Here's how the part is built. I have some questions about the finished solid (model axes, mm). A direction names the side the tool comes from. Give positions to 0.01 mm unless a question says otherwise; leave off trailing zeros. Write each loop counter-clockwise with the first axis right and the second up, starting at its lowest first coordinate (ties: lowest second). Pieces come first, ordered by that corner, then holes. Notation, with made-up numbers: (46, 13) - (51, 13) arc R24 cw to (51, 27) - close; hole circle Ø11 at (48, 47.25). An arc over 180 degrees is marked (long way). Use a Markdown table: item, result.
```python
from build123d import *
from OCP.BRepFilletAPI import BRepFilletAPI_MakeChamfer

# Parameters (mm, degrees)
EXTRUDE_1_DEPTH   = 0.32
EXTRUDE_1_2_DEPTH = 0.32
CHAMFER_1_SIZE    = 0.1
CHAMFER_1_SIZE2   = 0.274747742
FILLET_1_R        = 0.5
CHAMFER_2_SIZE    = 0.1
CHAMFER_2_SIZE2   = 0.274747742
FILLET_2_R        = 0.5
SKETCH_2_W        = 2.54
SKETCH_2_H        = 5
EXTRUDE_2_DEPTH   = 1.8
CHAMFER_3_SIZE    = 0.5
CHAMFER_4_SIZE    = 0.25
EXTRUDE_3_DEPTH   = 0.7


with BuildPart() as part:
    # Sketch 1 → Extrude 1 (new, symmetric)
    with BuildSketch(Plane(origin=(0, 0, 0), x_dir=(0, 0, -1), z_dir=(1, 0, 0))):
        Polygon((-0.7385, 0), (0.7385, 0), (0.7385, 0.64), (-0.47340332, 0.64), (-1.38340332, 1.55), (-11.4615, 1.55), (-11.4615, 0.91), (-1.6485, 0.91), align=None)
    extrude(amount=EXTRUDE_1_DEPTH, both=True)

    # Chamfer 2: one chamfer whose edges measure the first distance from different faces: ONE call of the kernel's chamfer builder (chamfer() names one face for all edges)
    chamfer_2_edges_1 = [part.edges().sort_by_distance(p)[0] for p in [
        (0.32, 0.32, -0.7385),
        (0, 0, -0.7385),
        (0, 0.64, -0.7385),
        (-0.32, 0.32, -0.7385),
    ]]
    chamfer_2_side_1 = [part.faces().sort_by_distance(p)[0] for p in [
        (0, 0.32, -0.7385),
    ]]
    chamfer_2_edges_2 = [part.edges().sort_by_distance(p)[0] for p in [
        (0, 0.91, 11.4615),
        (0, 1.55, 11.4615),
        (-0.32, 1.23, 11.4615),
        (0.32, 1.23, 11.4615),
    ]]
    chamfer_2_side_2 = [part.faces().sort_by_distance(p)[0] for p in [
        (0, 1.23, 11.4615),
    ]]
    chamfer_2 = BRepFilletAPI_MakeChamfer(part.part.solid().wrapped)
    for e in chamfer_2_edges_1:
        chamfer_2.Add(CHAMFER_2_SIZE, CHAMFER_2_SIZE2, e.wrapped, chamfer_2_side_1[0].wrapped)  # the first distance lies on this face
    for e in chamfer_2_edges_2:
        chamfer_2.Add(CHAMFER_2_SIZE, CHAMFER_2_SIZE2, e.wrapped, chamfer_2_side_2[0].wrapped)  # the first distance lies on this face
    add(Compound.cast(chamfer_2.Shape()), mode=Mode.REPLACE)

    # Fillet 2
    fillet_2_edges = [part.edges().sort_by_distance(p)[0] for p in [
        (0, 0, 0.7385),
        (0, 0.91, 1.6485),
        (0, 1.55, 1.38340332),
        (0, 0.64, 0.47340332),
    ]]
    fillet(fillet_2_edges, radius=FILLET_2_R)



with BuildPart() as body_2:
    # Sketch 1 → Extrude 1 2 (new, symmetric)
    with BuildSketch(Plane(origin=(0, 0, 0), x_dir=(0, 0, -1), z_dir=(1, 0, 0))):
        Polygon((4.0615, 0), (5.5385, 0), (5.5385, 0.64), (4.32659668, 0.64), (0.87659668, 4.09), (-11.4615, 4.09), (-11.4615, 3.45), (0.6115, 3.45), align=None)
    extrude(amount=EXTRUDE_1_2_DEPTH, both=True)

    # Chamfer 1: one chamfer whose edges measure the first distance from different faces: ONE call of the kernel's chamfer builder (chamfer() names one face for all edges)
    chamfer_1_edges_1 = [body_2.edges().sort_by_distance(p)[0] for p in [
        (-0.32, 0.32, -5.5385),
        (0, 0.64, -5.5385),
        (0, 0, -5.5385),
        (0.32, 0.32, -5.5385),
    ]]
    chamfer_1_side_1 = [body_2.faces().sort_by_distance(p)[0] for p in [
        (0, 0.32, -5.5385),
    ]]
    chamfer_1_edges_2 = [body_2.edges().sort_by_distance(p)[0] for p in [
        (0, 3.45, 11.4615),
        (0, 4.09, 11.4615),
        (-0.32, 3.77, 11.4615),
        (0.32, 3.77, 11.4615),
    ]]
    chamfer_1_side_2 = [body_2.faces().sort_by_distance(p)[0] for p in [
        (0, 3.77, 11.4615),
    ]]
    chamfer_1 = BRepFilletAPI_MakeChamfer(body_2.part.solid().wrapped)
    for e in chamfer_1_edges_1:
        chamfer_1.Add(CHAMFER_1_SIZE, CHAMFER_1_SIZE2, e.wrapped, chamfer_1_side_1[0].wrapped)  # the first distance lies on this face
    for e in chamfer_1_edges_2:
        chamfer_1.Add(CHAMFER_1_SIZE, CHAMFER_1_SIZE2, e.wrapped, chamfer_1_side_2[0].wrapped)  # the first distance lies on this face
    add(Compound.cast(chamfer_1.Shape()), mode=Mode.REPLACE)

    # Fillet 1
    fillet_1_edges = [body_2.edges().sort_by_distance(p)[0] for p in [
        (0, 3.45, -0.6115),
        (0, 4.09, -0.87659668),
        (0, 0.64, -4.32659668),
        (0, 0, -4.0615),
    ]]
    fillet(fillet_1_edges, radius=FILLET_1_R)


with BuildPart() as part_1:
    add(part.part)

    add(body_2.part)  # Extrude 2 merges body 2
    # Sketch 2 → Extrude 2 (add)
    with BuildSketch(Plane.XY.offset(3.661)):
        with Locations((0, 2.5)):
            Rectangle(SKETCH_2_W, SKETCH_2_H)
    extrude(amount=EXTRUDE_2_DEPTH)

    # Chamfer 3
    chamfer_3_edges = [part_1.edges().sort_by_distance(p)[0] for p in [
        (1.27, 0, 4.561),
        (1.27, 5, 4.561),
        (-1.27, 5, 4.561),
        (-1.27, 0, 4.561),
    ]]
    chamfer(chamfer_3_edges, length=CHAMFER_3_SIZE)

    # Chamfer 4
    chamfer_4_edges = [part_1.edges().sort_by_distance(p)[0] for p in [
        (-1.27, 2.5, 5.461),
        (1.27, 2.5, 5.461),
    ]]
    chamfer(chamfer_4_edges, length=CHAMFER_4_SIZE)

    # Sketch 3 → Extrude 3 (add)
    with BuildSketch(Plane(origin=(0, 0, 3.661), x_dir=(-1, 0, 0), z_dir=(0, 0, -1))):
        Polygon((-1.27, 4.5), (-0.77, 5), (0.77, 5), (1.27, 4.5), (1.27, 4.4), (-1.27, 4.4), align=None)
        Polygon((-1.27, 0.6), (-1.27, 0.5), (-0.77, 0), (0.77, 0), (1.27, 0.5), (1.27, 0.6), align=None)
    extrude(amount=EXTRUDE_3_DEPTH)


solid = part_1.part
```
Item 1: For faces 1 (the flat face through (0.32, 1.1, 1.6)), 2 (the flat face through (-0.32, 1.1, 1.6)), 3 (the flat face through (0, 0, 4)), which set-ups out of +Z, -Z, +X, -X, +Y, -Y let a thin tool reach every point of the face, with its end or its side?
Values:
| item | result |
|---|---|
| face 1 | -Z, +X |
| face 2 | -Z, -X |
| face 3 | +Z, -Z, +X, -X, -Y |
Item 2: If we section it at B-B, the plane y = 3.05: Write out the boundary of the cut face in (x, z).
Values:
| item | result |
|---|---|
| outline | (-1.27, 3.66) - (1.27, 3.66) - (1.27, 5.21) - (1.02, 5.46) - (-1.02, 5.46) - (-1.27, 5.21) - close; (-0.32, -1.92) - (0.32, -1.92) - (0.32, -1.01) - (-0.32, -1.01) - close |
Item 3: Thinking about a two-plate mould opening in Z: for faces 4 (the flat face through (0, 1.75, -2.31)), 5 (the flat face through (0.004, 2.343, -2.624)), 6 (the flat face through (-1.27, 3, 5)), which applies, +Z half, -Z half, draft (parallel to the pull), parting line (faces both ways), or undercut?
Values:
| item | result |
|---|---|
| face 4 | undercut |
| face 5 | -Z half |
| face 6 | draft |
Item 4: If we section it at A-A, the plane z = 6.75: Write out the boundary of the cut face in (x, y), plus the area to 3 significant figures.
Values:
| item | result |
|---|---|
| outline | (-0.32, 0.91) - (0.32, 0.91) - (0.32, 1.55) - (-0.32, 1.55) - close; (-0.32, 3.45) - (0.32, 3.45) - (0.32, 4.09) - (-0.32, 4.09) - close |
| area | 0.819 mm2 |
Item 5: I need wall thicknesses on line 1 along Z through (x, y) = (-0.45, 1.65); line 2 along X through (y, z) = (3.85, 10); line 3 along Y through (x, z) = (-0.05, 1.5). Which ranges of each line are inside material? Lowest first, please. Write a range as [from, to].
Values:
| item | result |
|---|---|
| line 1 | z = [3.66, 5.46] |
| line 2 | x = [-0.32, 0.32] |
| line 3 | y = [0.76, 1.54], [3.45, 4.09] |
Item 6: If we section it at D-D, the plane z = -2.75: Write out the boundary of the cut face in (x, y), plus the area to 3 significant figures.
Values:
| item | result |
|---|---|
| outline | (-0.32, 1.31) - (0.32, 1.31) - (0.32, 2.22) - (-0.32, 2.22) - close |
| area | 0.579 mm2 |
Item 7: Will these pins go through, and if not, where does the flat tip stop? pin 1 Ø0.7 at (x, z) = (0, 0) entering from +Y; pin 2 Ø1.3 at (x, y) = (0, 1.5) entering from -Z; pin 3 Ø0.7 at (x, y) = (0.5, 4.5) entering from -Z.
Values:
| item | result |
|---|---|
| pin 1 | stops at y = 4.09 |
| pin 2 | stops at z = -4.12 |
| pin 3 | stops at z = 2.96 |
Item 8: If we section it at C-C, the plane x = -0.5: Write out the boundary of the cut face in (y, z).
Values:
| item | result |
|---|---|
| outline | (0, 2.96) - (0.6, 2.96) - (0.6, 3.66) - (4.4, 3.66) - (4.4, 2.96) - (5, 2.96) - (5, 5.46) - (0, 5.46) - close |
